Check sheet for the modelled part. Datum: model origin and axes. Units: mm. A direction names the side the tool comes from. Give positions to 0.01 mm unless a question says otherwise; leave off trailing zeros. Order: outer loops, then holes, each group sorted by start corner. A loop starts at its lowest first (then second) coordinate and runs counter-clockwise, first axis right, second up.
Autodesk Inventor part; units mm, degrees
ref_plane "YZ Plane" through (0, 0, 0) normal (1, 0, 0) x (0, 1, 0)
ref_plane "XZ Plane" through (0, 0, 0) normal (0, 1, 0) x (-1, 0, 0)
ref_plane "XY Plane" through (0, 0, 0) normal (0, 0, 1) x (1, 0, 0)
sketch "Sketch1" plane through (0, 0, 0) normal (0, 1, 0) x (-1, 0, 0)
  line L0 (0, 0) -> (0, -16)
  line L1 (0, -16) -> (-13, -16)
  circle A0 centre (48.4003, -12.7173) radius 1
  circle A1 centre (48.4003, 5.2827) radius 1
  line L2 (0, 0) -> (-13, 0)
  line L3 (-16, 0) -> (-16, 1.0033)
  line L4 (-16, -16) -> (-16, -17.0033)
  circle A2 centre (-16, 1.0033) radius 1
  circle A3 centre (-16, -17.0033) radius 1
  arc A4 (-18.8273, -16) -> (-13.1727, -16) centre (-16, -17.0033) ccw
  arc A5 (-13.1727, 0) -> (-18.8273, 0) centre (-16, 1.0033) ccw
  line L5 (-19, 0) -> (-29.5, 0)
  line L6 (-19, -16) -> (-29.5, -16)
  line L7 (-29.5, 0) -> (-29.5, -16)
  line L8 (-29.5, -8) -> (-29.5, -19.65)
  line L9 (-29.5, -8) -> (-29.5, 3.6592)
  line L10 (-29.5, 3.6592) -> (-17.3951, 3.6592)
  line L11 (-29.5, -19.65) -> (-17.4124, -19.65)
  line L12 (-13, 0) -> (-13.1727, 0)
  line L13 (-18.8273, 0) -> (-19, 0)
  line L14 (-13, -16) -> (-13.1727, -16)
  line L15 (-18.8273, -16) -> (-19, -16)
  dimension "d0" = 16
  dimension "d1" = 13
  dimension "d2" = 6
  dimension "d3" = 1.0033
  dimension "d4" = 1.0033
  dimension "d5" = 2
  dimension "d6" = 2
  dimension "d7" = 6
  dimension "d8" = 6
  dimension "d9" = 6
  dimension "d10" = 13
  dimension "d11" = 10.5
  dimension "d12" = 11.65
extrude "Extrusion1" add sketch "Sketch1" along normal blind 0.65 contours L0 L1 L14 A4 L15 L6 L7 L5 L13 A5 L12 L2 | A5 L13 L5 L9 L10 | L11 L8 L6 L15 A4
sketch "Sketch2" plane through (0, 0.65, 0) normal (0, 1, 0) x (1, 0, 0)
  line L0 (0, 0) -> (13.1727, 0)
  circle A0 centre (16, -1.0033) radius 1
  circle A1 centre (16, 17.0033) radius 1
  line L1 (17.3951, -3.6592) -> (29.5, -3.6592)
  line L2 (29.5, -3.6592) -> (29.5, 19.65)
  line L3 (29.5, 19.65) -> (17.4124, 19.65)
  arc A2 (17.4124, 19.65) -> (13.1727, 16) centre (16, 17.0033) ccw
  line L4 (13.1727, 16) -> (0, 16)
  line L5 (0, 16) -> (0, 0)
  line L6 (0, 0) -> (13.1727, 0)
  arc A3 (13.1727, 0) -> (17.3951, -3.6592) centre (16, -1.0033) ccw
  line L7 (0, 0) -> (1.5, 0)
  line L8 (1.5, 0) -> (1.5, 2)
  line L9 (1.5, 2) -> (0, 2)
  line L10 (0, 2) -> (0, 0)
  line L11 (1.5, 2) -> (4, 2)
  line L12 (4, 2) -> (4, 5.5)
  line L13 (4, 5.5) -> (1.5, 5.5)
  line L14 (1.5, 5.5) -> (1.5, 2)
  line L15 (4, 2) -> (6, 2)
  line L16 (4, 2) -> (6, 2) construction
  line L17 (6, 2) -> (6, 5.5)
  line L18 (6, 5.5) -> (9.5052, 5.5)
  line L19 (6, 2) -> (9.5052, 2)
  line L20 (9.5052, 2) -> (9.5052, 5.5)
  line L21 (9.5052, 5.5) -> (6, 5.5)
  line L22 (6, 5.5) -> (6, 2)
  circle A4 centre (28.0254, -2.0033) radius 0.5
  circle A5 centre (26.5254, -2.0033) radius 0.5
  line L23 (26.5254, -2.0033) -> (28.0254, -2.0033)
  line L24 (26.5254, -2.0033) -> (25.0254, -2.0033)
  circle A6 centre (25.0254, -2.0033) radius 0.5
  line L25 (29.5, 7.9954) -> (27.2754, 7.9954)
  line L26 (1.5, 15.9908) -> (1.5, 13.9908)
  line L27 (1.5, 13.9908) -> (0, 13.9908)
  line L28 (1.5, 13.9908) -> (4, 13.9908)
  line L29 (4, 13.9908) -> (4, 10.4908)
  line L30 (4, 10.4908) -> (1.5, 10.4908)
  line L31 (1.5, 10.4908) -> (1.5, 13.9908)
  line L32 (4, 13.9908) -> (6, 13.9908)
  line L33 (4, 13.9908) -> (6, 13.9908) construction
  line L34 (6, 13.9908) -> (6, 10.4908)
  line L35 (6, 10.4908) -> (9.5052, 10.4908)
  line L36 (6, 13.9908) -> (9.5052, 13.9908)
  line L37 (9.5052, 13.9908) -> (9.5052, 10.4908)
  line L38 (9.5052, 10.4908) -> (6, 10.4908)
  line L39 (6, 10.4908) -> (6, 13.9908)
  circle A7 centre (28.0254, 17.9941) radius 0.5
  circle A8 centre (26.5254, 17.9941) radius 0.5
  line L40 (26.5254, 17.9941) -> (28.0254, 17.9941)
  line L41 (26.5254, 17.9941) -> (25.0254, 17.9941)
  circle A9 centre (25.0254, 17.9941) radius 0.5
  line L42 (1.893, 6.5402) -> (3.725, 6.5402)
  line L43 (3.725, 6.5402) -> (3.725, 9.4507)
  line L44 (3.725, 9.4507) -> (1.893, 9.4507)
  line L45 (1.893, 9.4507) -> (1.893, 6.5402)
  dimension "d15" = 1.5
  dimension "d16" = 2
  dimension "d17" = 2.5
  dimension "d18" = 3.5
  dimension "d19" = 2
  dimension "d20" = 0
  dimension "d21" = 3.5052
  dimension "d22" = 90
  dimension "d23" = 1
  dimension "d24" = 1
  dimension "d25" = 1.5
  dimension "d26" = 1.5
  dimension "d27" = 1
  dimension "d33" = 1.0402
  dimension "d34" = 1.0402
extrude "Extrusion2" add sketch "Sketch2" along normal blind 1.7 contours L14 L13 L12 L11 | L17 L18 L20 L19 | A4 | L23 L24 A5 | A5 L24 L23 | A6 | L28 L29 L30 L31 | L36 L37 L35 L34 | A7 | L40 L41 A8 | A8 L41 L40 | A9 | L45 L44 L43 L42
chamfer "Chamfer1" distance 0.5 angle 45 6 edges at (27.5254, 2.35, -17.9941) (26.0254, 2.35, -17.9941) (24.5254, 2.35, -17.9941) (27.5254, 2.35, 2.0033) (26.0254, 2.35, 2.0033) (24.5254, 2.35, 2.0033)
sketch "Sketch3" plane through (0, 0, 0) normal (0, -1, 0) x (1, 0, 0)
  circle A0 centre (16, -17.0033) radius 1
  circle A1 centre (16, 1.0033) radius 1
  line L0 (29.5, 3.6592) -> (29.5, -19.65)
  line L1 (17.3951, 3.6592) -> (29.5, 3.6592)
  arc A2 (17.3951, 3.6592) -> (13.1727, 0) centre (16, 1.0033) ccw
  line L2 (0, 0) -> (13.1727, 0)
  line L3 (0, -16) -> (0, 0)
  line L4 (13.1727, -16) -> (0, -16)
  arc A3 (13.1727, -16) -> (17.4124, -19.65) centre (16, -17.0033) ccw
  line L5 (29.5, -19.65) -> (17.4124, -19.65)
  line L6 (0, -16) -> (8, -16)
  line L7 (8, -16) -> (8, -11.3)
  line L8 (8, -11.3) -> (0, -11.3)
  line L9 (0, -11.3) -> (0, -16)
  line L10 (0, -16) -> (0, 0)
  line L11 (0, -8) -> (1.7097, -8)
  line L12 (0, 0) -> (0, -16)
  line L13 (13.1727, 0) -> (0, 0)
  line L14 (0, 0) -> (8, 0)
  line L15 (8, 0) -> (8, -4.7)
  line L16 (8, -4.7) -> (0, -4.7)
  line L17 (0, -4.7) -> (0, 0)
  line L18 (0, 0) -> (0, -16)
  line L19 (29.5, 3.6592) -> (29.5, -19.65)
  line L20 (29.5, -19.65) -> (21.5, -19.65)
  line L21 (21.5, -19.65) -> (21.5, -14.95)
  line L22 (21.5, -14.95) -> (29.5, -14.95)
  line L23 (29.5, -14.95) -> (29.5, -19.65)
  line L24 (29.5, 3.6592) -> (21.5, 3.6592)
  line L25 (21.5, 3.6592) -> (21.5, -1.0408)
  line L26 (21.5, -1.0408) -> (29.5, -1.0408)
  line L27 (29.5, -1.0408) -> (29.5, 3.6592)
  dimension "d35" = 8
  dimension "d36" = 4.7
  dimension "d39" = 8
  dimension "d40" = 4.7
  dimension "d41" = 8
  dimension "d42" = 4.7
extrude "Extrusion3" add sketch "Sketch3" along normal blind 6 contours L0 L26 L25 L1 | L0 L5 L21 L22
equation "\"d34\" = d33"
properties part number "Encoder"
(1) Go/stop test with flat-tipped pins: P1, Ø0.5, axis at y = 2, z = -4, coming from the -X side; P2, Ø0.5, axis at x = 2.5, y = 1, coming from the +Z side; P3, Ø8, axis at x = 13, z = -10, coming from the -Y side; P4, Ø1.2, axis at x = 16, z = 1, coming from the +Y side. Record where each tip stops, or that it passes through.
(2) Sectioned sample at B-B (y = -1.75). Enter the section's corners in (x, z).
(3) Thickness scan on L1, parallel to Z at x = 23, y = -4.5; L2, parallel to Z at x = 16, y = 0.3; L3, parallel to Y at x = 13, z = -7.5. Record the ranges inside material, lowest first.
(4) Tool access check on faces 4 (the face through (6, 1, -12)), 5 (the face through (3.725, 1, -8)), 6 (the face through (25, -3, -1.041)), 7 (the face through (8, 1, -2)). Record the directions out of +Z, -Z, +X, -X, +Y, -Y that give a thin tool (end or side, any length) a straight path to the whole face; none if there is none.
(5) Release check for a two-part mould opening along X. For faces 1 (the face through (25, -3, -19.65)), 2 (the face through (21.5, -3, 1)), 3 (the face through (26.417, 1.242, 1.515)) record: released by +X, released by -X, zero draft, split by the parting line, or undercut.
(6) Sectioned sample at D-D (z = -3.5). Enter the section's corners in (x, y), plus the area to 3 significant figures.
(7) Sectioned sample at A-A (x = 16). Enter the section's corners in (y, z).
(8) Sectioned sample at C-C (y = 1.25). Count the separate pieces of the cut face and the enclosed holes in it, plus the area to 3 significant figures.
Values follow:
1. P1: stops at x = 1.5
1. P2: stops at z = -2
1. P3: stops at y = 0
1. P4: passes through
2. outline: (21.5, -19.65) - (29.5, -19.65) - (29.5, -14.95) - (21.5, -14.95) - close; (21.5, -1.04) - (29.5, -1.04) - (29.5, 3.66) - (21.5, 3.66) - close
3. L1: z = -19.65 to -14.95, -1.04 to 3.66
3. L2: z = -20 to -18, -16 to 0, 2 to 4
3. L3: y = 0 to 0.65
4. face 4: +Z, -Z, +Y
4. face 5: +X, +Y
4. face 6: +X, -X, -Y
4. face 7: +Z, +X, -X, +Y
5. face 1: zero draft
5. face 2: released by -X
5. face 3: undercut
6. outline: (0, 0) - (29.5, 0) - (29.5, 0.65) - (9.51, 0.65) - (9.51, 2.35) - (6, 2.35) - (6, 0.65) - (4, 0.65) - (4, 2.35) - (1.5, 2.35) - (1.5, 0.65) - (0, 0.65) - close
6. area: 29.4 mm2
7. outline: (0, -20) - (0.65, -20) - (0.65, -18) - (0, -18) - close; (0, -16) - (0.65, -16) - (0.65, 0) - (0, 0) - close; (0, 2) - (0.65, 2) - (0.65, 4) - (0, 4) - close
8. separate pieces: 11
8. enclosed holes: 0
8. area: 52.1 mm2
